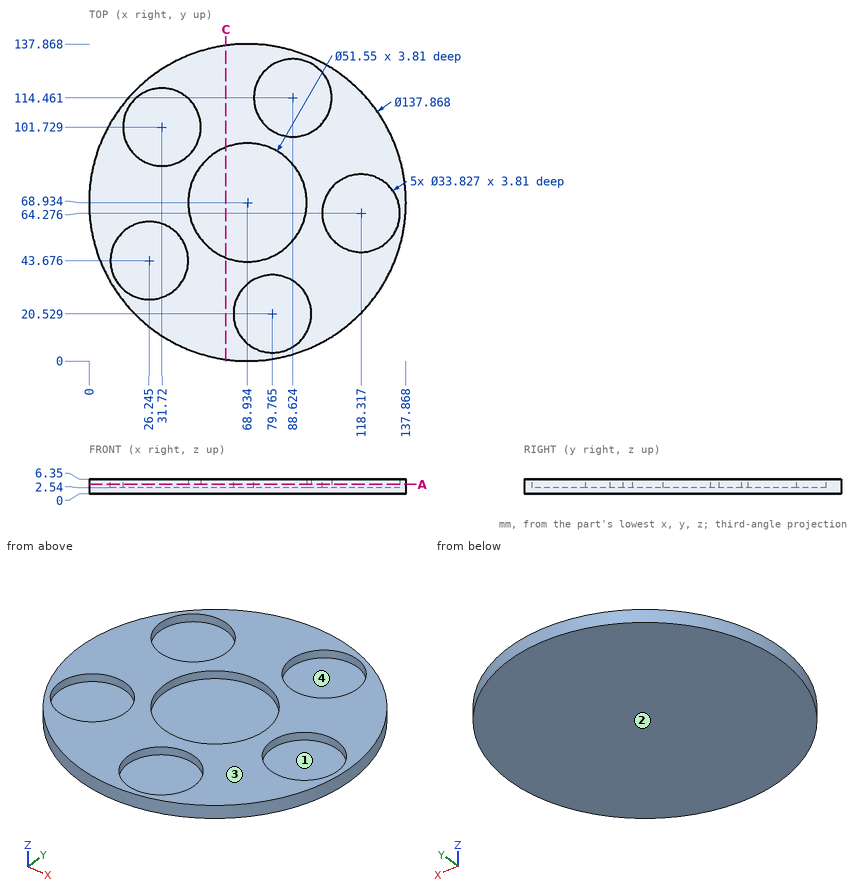
The figure shows three views and two pictorial views of one solid part (mm, origin at its lowest corner). Answer the questions. A direction names the side the tool comes from. Give positions to 0.01 mm unless a question says otherwise; leave off trailing zeros. Write each loop counter-clockwise with the first axis right and the second up, starting at its lowest first coordinate (ties: lowest second). Pieces come first, ordered by that corner, then holes. Notation, with made-up numbers: (54.5, 48.25) - (69.5, 48.25) arc R26 cw to (69.5, 63.25) - close; hole circle Ø5 at (-17.75, 31). An arc over 180 degrees is marked (long way). Use CSV: the item, a comma, the result in double quotes. Start each with the question number.
Item 1: Consider line 1 (X direction, y = 28, z = 4.75) (1 decimal); line 2 (X direction, y = 57.5, z = 3.5) (1 decimal); line 3 (Z direction, x = 109.5, y = 72.5). Determine where each line is inside the solid, lowest interval first.
Item 2: Flat-ended cylindrical pins translate along their axes: P1, Ø1, axis at y = 122.5, z = 3, coming from the -X side (1 decimal); P2, Ø1, axis at y = 16.5, z = 3.5, coming from the -X side (1 decimal); P3, Ø1, axis at x = 91.5, y = 76, coming from the +Z side. Find the tip coordinate at first contact, or state that the pin passes through.
Item 3: The mould has two halves that part along X. Classify the marked faces 1 and 2: pulls with the +X half, pulls with the -X half, needs draft (parallel to the pull), parting line crosses it, or undercut.
Item 4: For the marked faces 3 and 4, determine the directions among +Z, -Z, +X, -X, +Y, -Y from which every point of the face is accessible in a straight line to the end or side of a thin tool.
Item 5: The part is cut by section A-A, the plane z = 4. Count the separate pieces of the cut face and the enclosed holes in it, and give its area (3 significant figures).
Item 6: The part is cut by section C-C, the plane x = 59.5. Give the vertices of the cut face in (y, z).
Taken from the geometry:
1,line 1,"13.5 to 19.9, 32.6 to 64.6, 94.9 to 124.4"
1,line 2,"1 to 16.5, 36 to 45.8, 92 to 102.8, 133.8 to 136.9"
1,line 3,"0 to 2.54"
2,P1,"x = 24.9"
2,P2,"x = 23.6"
2,P3,"z = 2.54"
3,face 1,"undercut"
3,face 2,"needs draft"
4,face 3,"+Z, +X, -X, +Y, -Y"
4,face 4,"+Z"
5,separate pieces,"1"
5,enclosed holes,"6"
5,area,"8,350 mm2"
6,outline,"(0.65, 0) - (137.22, 0) - (137.22, 6.35) - (92.92, 6.35) - (92.92, 2.54) - (44.95, 2.54) - (44.95, 6.35) - (0.65, 6.35) - close"
